Read the model definition and answer for the solid it produces. Units are mm, in the model's axes. Face numbers are marked on the shaded views. A direction names the side the tool comes from. Coordinates: 2 decimals unless noted, no trailing zeros. Order: outer loops, then holes, each group sorted by start corner. A loop starts at its lowest first (then second) coordinate and runs counter-clockwise, first axis right, second up.
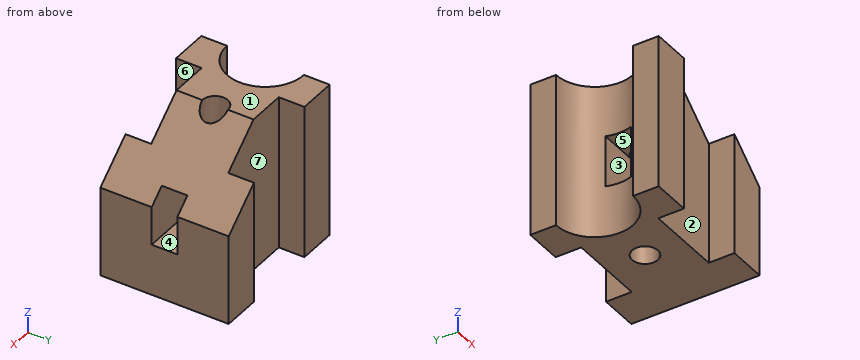
```python
from build123d import *

# Parameters (mm, degrees)
SKETCH1_R           = 5
BOSS_EXTRUDE1_DEPTH = 60
CUT_EXTRUDE3_DEPTH  = 60
SKETCH7_W           = 20
SKETCH7_H           = 10
CUT_EXTRUDE4_DEPTH  = 60


with BuildPart() as part:
    # Sketch1 → Boss-Extrude1 (new body)
    with BuildSketch(Plane.XY):
        with BuildLine():
            Line((-23.203125, -22.890625), (-23.203125, -32.890625))
            Line((-23.203125, -32.890625), (-38.203125, -32.890625))
            Line((-38.203125, -32.890625), (-38.203125, -22.890625))
            ThreePointArc((-38.203125, -22.890625), (-23.203125, -7.890625), (-38.203125, 7.109375))
            Line((-38.203125, 7.109375), (-38.203125, 17.109375))
            Line((-38.203125, 17.109375), (-23.203125, 17.109375))
            Line((-23.203125, 17.109375), (-23.203125, 7.109375))
            Line((-23.203125, 7.109375), (6.796875, 7.109375))
            Line((6.796875, 7.109375), (6.796875, 17.109375))
            Line((6.796875, 17.109375), (21.796875, 17.109375))
            Line((21.796875, 17.109375), (21.796875, -32.890625))
            Line((21.796875, -32.890625), (6.796875, -32.890625))
            Line((6.796875, -32.890625), (6.796875, -22.890625))
            Line((6.796875, -22.890625), (-23.203125, -22.890625))
        make_face()
        with Locations((-8.203125, -7.890625)):
            Circle(SKETCH1_R, mode=Mode.SUBTRACT)
    extrude(amount=BOSS_EXTRUDE1_DEPTH)

    # Sketch3 → Cut-Extrude3 (cut)
    with BuildSketch(Plane(origin=(0, 17.109375, 0), x_dir=(1, 0, 0), z_dir=(0, 1, 0))):
        Polygon((-8.203125, -60), (21.796875, -35), (21.796875, -60), align=None)
    extrude(amount=-CUT_EXTRUDE3_DEPTH, mode=Mode.SUBTRACT)

    # Sketch7 → Cut-Extrude4 (cut)
    with BuildSketch(Plane(origin=(21.796875, 0, 0), x_dir=(0, 0, -1), z_dir=(1, 0, 0))):
        with Locations((-30, -7.890625)):
            Rectangle(SKETCH7_W, SKETCH7_H)
    extrude(amount=-CUT_EXTRUDE4_DEPTH, mode=Mode.SUBTRACT)


solid = part.part
```
1) Which of the six approach directions +Z, -Z, +X, -X, +Y, -Y give full straight-line access (tool end or side, diameter ignored) to the marked faces 5, 6 and 7?
A:
face 5: +X, -X
face 6: +Z, -Z, -Y
face 7: +Z, -Z, +Y
2) Straight lines are drawn through the part: line 1 (Y direction, x = -4.5, z = 32.5); line 2 (X direction, y = -23.5, z = 23); line 3 (Y direction, x = -25.5, z = 25). For each, find the intervals that lie inside material, in ascending order.
A:
line 1: y = -22.89 to -12.89, -2.89 to 7.11
line 2: x = -38.2 to -23.2, 6.8 to 21.8
line 3: y = -32.89 to -15.87, 0.09 to 17.11
3) A cutting plane is placed at D-D, the plane x = -29. Determine the outline of the cut face in (y, z).
A:
outline: (-32.89, 0) - (-19.74, 0) - (-19.74, 60) - (-32.89, 60) - close; (3.95, 0) - (17.11, 0) - (17.11, 60) - (3.95, 60) - close
4) A cutting plane is placed at C-C, the plane z = 42. Determine the outline of the cut face in (x, y).
A:
outline: (-38.2, -32.89) - (-23.2, -32.89) - (-23.2, -22.89) - (6.8, -22.89) - (6.8, -32.89) - (13.4, -32.89) - (13.4, 17.11) - (6.8, 17.11) - (6.8, 7.11) - (-23.2, 7.11) - (-23.2, 17.11) - (-38.2, 17.11) - (-38.2, 7.11) arc R15 cw to (-38.2, -22.89) - close; hole circle Ø10 at (-8.2, -7.89)
5) Flat-ended cylindrical pins translate along their axes: pin 1 Ø22 at (x, z) = (-7, 27.5) entering from +Y; pin 2 Ø11 at (x, y) = (0.5, -7.5) entering from +Z; pin 3 Ø3 at (x, z) = (-7, 7) entering from -Y. Find the tip coordinate at first contact, or state that the pin passes through.
A:
pin 1: stops at y = 7.11
pin 2: stops at z = 56.73
pin 3: stops at y = -22.89
6) A cutting plane is placed at A-A, the plane y = 10.5. Determine the outline of the cut face in (x, z), and give its area (3 significant figures).
A:
outline: (-38.2, 0) - (-23.2, 0) - (-23.2, 60) - (-38.2, 60) - close; (6.8, 0) - (21.8, 0) - (21.8, 35) - (6.8, 47.5) - close
area: 1,520 mm2
7) Determine the mould class of the marked faces 1, 2, 3 and 4 for opening direction Y: pulls with the +Y half, pulls with the -Y half, needs draft (parallel to the pull), parting line crosses it, or undercut.
A:
face 1: needs draft
face 2: pulls with the -Y half
face 3: undercut
face 4: undercut
8) A cutting plane is placed at B-B, the plane x = -22. Determine the outline of the cut face in (y, z).
A:
outline: (-22.89, 0) - (7.11, 0) - (7.11, 60) - (-22.89, 60) - close; hole (-12.89, 20) - (-2.89, 20) - (-2.89, 40) - (-12.89, 40) - close
